Here's how the part is built. I have some questions about the finished solid (model axes, mm). A direction names the side the tool comes from. Give positions to 0.01 mm unless a question says otherwise; leave off trailing zeros. Loops run counter-clockwise (first coordinate to the right, second up) from the corner with the lowest first, then second, coordinate; pieces in that order, holes last.
Q1. Will these pins go through, and if not, where does the flat tip stop? P1, Ø2.5, axis at x = 1, z = 29.5, coming from the +Y side; P2, Ø6.5, axis at x = -2.5, z = -32, coming from the +Y side.
Q2. We'd pull the mould along X, two halves only. Please class faces 1 (the face through (0, 7, 1)), 2 (the face through (-8, 4, -49)), 3 (the face through (0.358, 1.232, -32.727)): +X half, -X half, draft (parallel to the pull), parting line (faces both ways), or undercut.
Q3. If we section it at C-C (x = -8): Please give me the cut outline in (y, z).
Q4. If we section it at A-A (x = 0): Please give me the cut outline in (y, z), plus the area to 3 significant figures.
Q5. If we section it at B-B (y = 4.5): Please give me the cut outline in (x, z).
Q6. I need wall thicknesses on line 1 (Z direction, x = 0, y = 1.05); line 2 (Z direction, x = 1, y = 5.75); line 3 (X direction, y = 1.7, z = -30). Which ranges of each line are inside material? Lowest first, please.
Q7. For faces 4 (the face through (0, 2.5, 27)), 5 (the face through (-10, 3, 1)), which set-ups out of +Z, -Z, +X, -X, +Y, -Y let a thin tool reach every point of the face, with its end or its side?
Autodesk Inventor part; units mm, degrees
ref_plane "YZ Plane" through (0, 0, 0) normal (1, 0, 0) x (0, 1, 0)
ref_plane "XZ Plane" through (0, 0, 0) normal (0, 1, 0) x (-1, 0, 0)
ref_plane "XY Plane" through (0, 0, 0) normal (0, 0, 1) x (1, 0, 0)
sketch "Sketch1" plane through (0, 0, 0) normal (0, 1, 0) x (-1, 0, 0)
  line L0 (-10, 50) -> (10, 50)
  line L1 (10, 50) -> (10, -50)
  line L2 (10, -50) -> (-10, -50)
  line L3 (-10, -50) -> (-10, 50)
  line L4 (-10, 50) -> (10, -50) construction
  line L5 (10, 50) -> (-10, -50) construction
  circle A0 centre (0, 30) radius 2.75
  circle A1 centre (0, -30) radius 2.75
  point P0 (0, 0)
  dimension "d0" = 20
  dimension "d1" = 100
  dimension "d2" = 5.5
  dimension "d3" = 20
  dimension "d4" = 20
extrude "Extrusion1" add sketch "Sketch1" along normal blind 7
sketch "Sketch2" plane through (0, 7, 0) normal (0, 1, 0) x (1, 0, 0)
  circle A0 centre (0, -30) radius 2.75
  circle A1 centre (0, -30) radius 4.1
  circle A2 centre (0, 30) radius 2.75
  circle A3 centre (0, 30) radius 4.1
  line L0 (-4.7343, -30) -> (-2.3671, -25.9)
  line L1 (-2.3671, -25.9) -> (2.3671, -25.9)
  line L2 (2.3671, -25.9) -> (4.7343, -30)
  line L3 (4.7343, -30) -> (2.3671, -34.1)
  line L4 (2.3671, -34.1) -> (-2.3671, -34.1)
  line L5 (-2.3671, -34.1) -> (-4.7343, -30)
  line L6 (-4.7343, 30) -> (-2.3671, 34.1)
  line L7 (-2.3671, 34.1) -> (2.3671, 34.1)
  line L8 (2.3671, 34.1) -> (4.7343, 30)
  line L9 (4.7343, 30) -> (2.3671, 25.9)
  line L10 (2.3671, 25.9) -> (-2.3671, 25.9)
  line L11 (-2.3671, 25.9) -> (-4.7343, 30)
  point P0 (0, 0)
  dimension "d7" = 8.2
extrude "Extrusion2" cut sketch "Sketch2" against normal blind 4.5 contours A0 | A1 | A1 L2 L3 | A1 L1 L2 | L3 L4 A1 | A1 L0 L1 | L4 L5 A1 | A1 L5 L0 | A2 | A3 | A3 L8 L9 | A3 L7 L8 | L9 L10 A3 | A3 L6 L7 | L10 L11 A3 | A3 L11 L6
fillet "Fillet1" radius 5 2 edges at (-10, 3.5, 50) (-10, 3.5, -50)
properties part number "Rubberplate2"
Check sheet entries:
1. P1: passes through
1. P2: stops at y = 7
2. face 1: draft
2. face 2: -X half
2. face 3: undercut
3. outline: (0, -49) - (7, -49) - (7, 49) - (0, 49) - close
4. outline: (0, -50) - (7, -50) - (7, -34.1) - (2.5, -34.1) - (2.5, -32.75) - (0, -32.75) - close; (0, -27.25) - (2.5, -27.25) - (2.5, -25.9) - (7, -25.9) - (7, 25.9) - (2.5, 25.9) - (2.5, 27.25) - (0, 27.25) - close; (0, 32.75) - (2.5, 32.75) - (2.5, 34.1) - (7, 34.1) - (7, 50) - (0, 50) - close
4. area: 599 mm2
5. outline: (-10, -45) arc R5 ccw to (-5, -50) - (10, -50) - (10, 50) - (-5, 50) arc R5 ccw to (-10, 45) - close; hole (-4.73, -30) - (-2.37, -34.1) - (2.37, -34.1) - (4.73, -30) - (2.37, -25.9) - (-2.37, -25.9) - close; hole (-4.73, 30) - (-2.37, 25.9) - (2.37, 25.9) - (4.73, 30) - (2.37, 34.1) - (-2.37, 34.1) - close
6. line 1: z = -50 to -32.75, -27.25 to 27.25, 32.75 to 50
6. line 2: z = -50 to -34.1, -25.9 to 25.9, 34.1 to 50
6. line 3: x = -10 to -2.75, 2.75 to 10
7. face 4: +Y
7. face 5: +Z, -Z, -X, +Y, -Y
